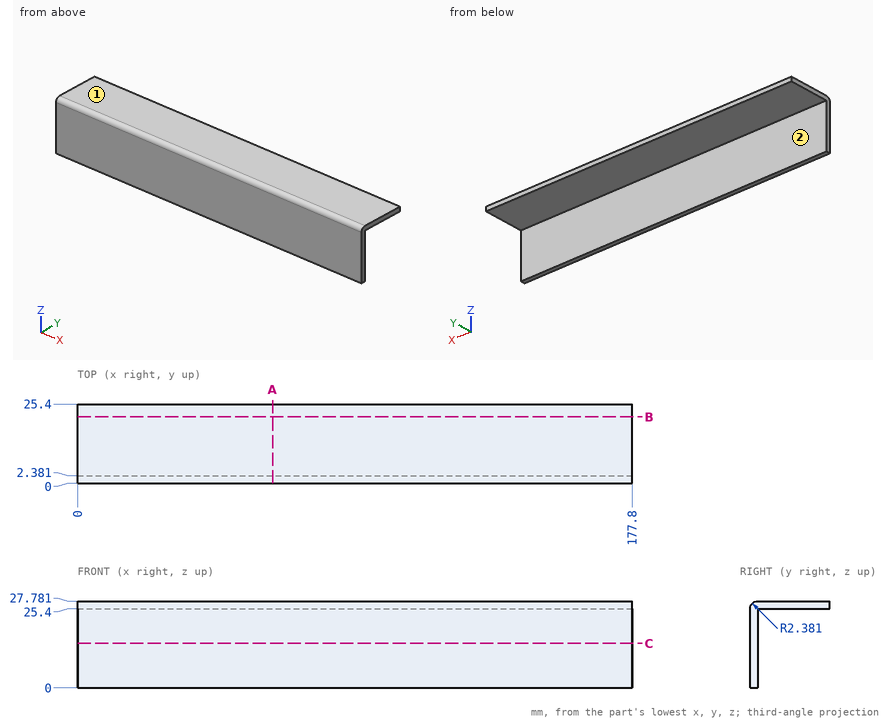
Job drawing, mm, ordinate dimensions from the low corner. One solid piece. A direction names the side the tool comes from. Coordinates: 2 decimals unless noted, no trailing zeros. Loops run counter-clockwise (first coordinate to the right, second up) from the corner with the lowest first, then second, coordinate; pieces in that order, holes last. Notation, with made-up numbers: (-39.75, 24) -> (5.25, 24) arc R30 cw to (5.25, 47) -> close; hole circle Ø3 at (63.5, -23). An arc over 180 degrees is marked (long way). One line per item, written item: value.
1. Drill centre lines: line 1 (Y direction, x = 28, z = 9); line 2 (Z direction, x = 54, y = 22); line 3 (Y direction, x = 46.5, z = 25.75). Where is each one in solid material? Low to high. Write a range as [from, to].
Answers:
line 1: y = [0, 2.38]
line 2: z = [25.4, 27.78]
line 3: y = [0.03, 25.4]
2. Flat gauge pins, fed straight in: P1, Ø1.5, axis at x = 104, y = 4, coming from the -Z side; P2, Ø7.5, axis at x = 84.5, z = 8.5, coming from the +Y side. Where does each tip first touch, or does it go through?
Answers:
P1: stops at z = 25.4
P2: stops at y = 2.38
3. Which spindle directions (+Z, -Z, +X, -X, +Y, -Y) get a long thin tool onto all of the face, cutting with end or side? Do the marked faces 1 and 2. Say none if no direction does.
Answers:
face 1: +Z, +X, -X, +Y, -Y
face 2: -Z, +X, -X, +Y
4. Slice it at A-A on x = 62.5. Write the cut outline in (y, z), and give its area (3 significant figures).
Answers:
outline: (0, 0) -> (2.38, 0) -> (2.38, 25.4) -> (25.4, 25.4) -> (25.4, 27.78) -> (2.38, 27.78) arc R2.38 ccw to (0, 25.4) -> close
area: 120 mm^2
5. Slice it at C-C on z = 14.25. Write the cut outline in (x, y).
Answers:
outline: (0, 0) -> (177.8, 0) -> (177.8, 2.38) -> (0, 2.38) -> close
6. Slice it at B-B on y = 21.25. Write the cut outline in (x, z).
Answers:
outline: (0, 25.4) -> (177.8, 25.4) -> (177.8, 27.78) -> (0, 27.78) -> close
